Autodesk Inventor part; units mm, degrees
ref_plane "YZ Plane" through (0, 0, 0) normal (1, 0, 0) x (0, 1, 0)
ref_plane "XZ Plane" through (0, 0, 0) normal (0, 1, 0) x (-1, 0, 0)
ref_plane "XY Plane" through (0, 0, 0) normal (0, 0, 1) x (1, 0, 0)
sketch "Sketch1" plane through (0, 0, 0) normal (0, 0, 1) x (1, 0, 0)
  line L0 (0, 25.4) -> (0, 0)
  line L1 (0, 0) -> (25.4, 0)
  line L2 (3.175, 25.4) -> (3.175, 4.953)
  line L3 (4.953, 3.175) -> (25.4, 3.175)
  line L4 (0, 25.4) -> (3.175, 25.4)
  line L5 (25.4, 3.175) -> (25.4, 0)
  line L6 (3.175, 4.953) -> (3.175, 3.175)
  line L7 (4.953, 3.175) -> (3.175, 3.175)
  dimension "d0" = 25.4
  dimension "d1" = 25.4
  dimension "d2" = 3.175
extrude "Extrusion1" add sketch "Sketch1" along normal blind 492.125
sketch "Sketch2" plane through (3.175, 3.175, 0) normal (0, 1, 0) x (1, 0, 0)
  circle A0 centre (9.525, -479.425) radius 2.8398
  line L0 (22.225, -492.125) -> (0, -492.125)
  line L1 (22.225, 0) -> (22.225, -492.125)
  circle A1 centre (9.525, -12.7) radius 2.8398
  line L2 (22.225, 0) -> (0, 0)
  point P0 (-3.175, 0)
  point P1 (1.778, -492.125)
  point P2 (1.778, 0)
  dimension "d5" = 12.7
  dimension "d6" = 12.7
  dimension "d9" = 466.725
  dimension "d31" = 12.7
hole "rail" at (12.7, 3.175, 479.425) at (12.7, 3.175, 12.7) direction (0, -1, 0) diameter 6.7564 depth 25.4 tip angle 118
sketch "Sketch7" plane through (3.175, 3.175, 0) normal (1, 0, 0) x (0, 0, -1)
  circle A0 centre (-479.425, 9.525) radius 2.8124
  line L0 (0, 22.225) -> (-492.125, 22.225)
  line L1 (-492.125, 0) -> (-492.125, 22.225)
  circle A1 centre (-12.7, 9.525) radius 2.8124
  point P0 (0, -3.175)
  dimension "d43" = 12.7
  dimension "d44" = 12.7
  dimension "d47" = 466.725
hole "mount" at (3.175, 12.7, 479.425) at (3.175, 12.7, 12.7) direction (-1, 0, 0) diameter 6.7564 depth 25.4 tip angle 118
sketch "Sketch8" plane through (3.175, 3.175, 0) normal (0, 1, 0) x (1, 0, 0)
  circle A0 centre (9.525, -479.425) radius 3.3782
  circle A1 centre (9.525, -12.7) radius 3.3782
  line L0 (9.525, -479.425) -> (9.525, -12.7) construction
  circle A2 centre (9.525, -246.0625) radius 3.3782
  point P0 (-3.175, 0)
hole "Hole5" at (12.7, 3.175, 246.0625) direction (0, -1, 0) diameter 6.7564 depth 25.4 tip angle 118
properties part number "angle_L11"
Work out the finished part from the listing and answer in its coordinate system (mm). A direction names the side the tool comes from. Coordinates: 2 decimals unless noted, no trailing zeros. Order: outer loops, then holes, each group sorted by start corner. A loop starts at its lowest first (then second) coordinate and runs counter-clockwise, first axis right, second up. Notation, with made-up numbers: M 40,-1 L 65,-1 A30 cw 65,28 Z; hole C 68.5,85 d10. An arc over 180 degrees is marked long. Use CSV: the item, a comma, the result in double quotes.
1) Consider line 1 (Z direction, x = 12.7, y = 2.5) (3 decimals); line 2 (Z direction, x = 1.8, y = 12.7) (3 decimals); line 3 (Y direction, x = 7.5, z = 72.5) (3 decimals). Determine where each line is inside the solid, lowest interval first. Write a range as [from, to].
Worked out:
line 1,"z = [0, 9.322], [16.078, 242.684], [249.441, 476.047], [482.803, 492.125]"
line 2,"z = [0, 9.322], [16.078, 476.047], [482.803, 492.125]"
line 3,"y = [0, 3.175]"
2) Flat-ended cylindrical pins translate along their axes: pin 1 Ø5.5 at (x, z) = (12.7, 479.425) entering from +Y; pin 2 Ø8 at (y, z) = (12.7, 12.7) entering from +X (3 decimals). Find the tip coordinate at first contact, or state that the pin passes through.
Worked out:
pin 1,"passes through"
pin 2,"stops at x = 3.175"
3) For faces 1 (the face through (15, 0, 243)), 2 (the face through (14.4, 3.175, 242.6)), determine the directions among +Z, -Z, +X, -X, +Y, -Y from which every point of the face is accessible in a straight line to the end or side of a thin tool.
Worked out:
face 1,"+Z, -Z, +X, -X, -Y"
face 2,"+Z, -Z, +X, +Y"
4) Section A-A on z = 300.5 is taken. Write down the section's boundary in (x, y) (3 decimals).
Worked out:
outline,"M 0,0 L 25.4,0 L 25.4,3.175 L 3.175,3.175 L 3.175,25.4 L 0,25.4 Z"
5) Section B-B on x = 21.5 is taken. Write down the section's boundary in (y, z) (3 decimals).
Worked out:
outline,"M 0,0 L 3.175,0 L 3.175,492.125 L 0,492.125 Z"
